Design review of the part built by this model. Coordinates are the model's own, in mm. Face numbers are marked on the shaded views. A direction names the side the tool comes from. Give positions to 0.01 mm unless a question says otherwise; leave off trailing zeros. Write each loop counter-clockwise with the first axis right and the second up, starting at its lowest first coordinate (ties: lowest second). Pieces come first, ordered by that corner, then holes. Notation, with made-up numbers: (55.25, -25.75) - (108.25, -25.75) arc R26 cw to (108.25, -5.75) - close; hole circle Ø11 at (16.5, -13.5). An arc over 180 degrees is marked (long way). Use a Markdown table: item, result. Add a question column.
```python
from build123d import *

# Parameters (mm, degrees)
F1_DEPTH = 101.6
F2_R     = 12.7
F3_DEPTH = 177.8
F4_R     = 7.9375
F4_R_2   = 6.35
F5_DEPTH = 177.8


with BuildPart() as f1:
    # F0 (on Front) → F1 (new body)
    with BuildSketch(Plane.XZ):
        with BuildLine():
            Line((-66.675, 136.525), (-66.675, 0))
            Line((-66.675, 0), (-60.325, 0))
            Line((-60.325, 0), (-60.325, 136.525))
            ThreePointArc((-60.325, 136.525), (-57.535192, 143.260192), (-50.8, 146.05))
            Line((-50.8, 146.05), (50.8, 146.05))
            ThreePointArc((50.8, 146.05), (57.535192, 143.260192), (60.325, 136.525))
            Line((60.325, 136.525), (60.325, 0))
            Line((60.325, 0), (66.675, 0))
            Line((66.675, 0), (66.675, 136.525))
            ThreePointArc((66.675, 136.525), (62.02532, 147.75032), (50.8, 152.4))
            Line((50.8, 152.4), (-50.8, 152.4))
            ThreePointArc((-50.8, 152.4), (-62.02532, 147.75032), (-66.675, 136.525))
        make_face()
    extrude(amount=F1_DEPTH)

    # F2 (on face) → F3 (join)
    with BuildSketch(Plane.XY.offset(152.4)):
        with Locations((0, -50.8)):
            Circle(F2_R)
    extrude(amount=F3_DEPTH)

    # F4 (on face) → F5 (cut)
    with BuildSketch(Plane.YZ.offset(66.675)):
        with BuildLine():
            Line((-101.6, 131.336227), (-101.6, 0))
            Line((-101.6, 0), (-25.4, 0))
            ThreePointArc((-25.4, 0), (-38.346191, 3.546942), (-47.676682, 13.197154))
            ThreePointArc((-47.676682, 13.197154), (-47.876619, 13.569464), (-48.070335, 13.945048))
            Line((-48.070335, 13.945048), (-94.291548, 101.759887))
            ThreePointArc((-94.291548, 101.759887), (-99.745816, 116.103258), (-101.6, 131.336227))
        make_face()
        with BuildLine():
            ThreePointArc((-48.070335, 13.945048), (-47.876619, 13.569464), (-47.676682, 13.197154))
            Line((-47.676682, 13.197154), (-48.070335, 13.945048))
        make_face()
        with Locations((-25.4, 25.4)):
            Circle(F4_R)
        with Locations((-50.8, 316.940695)):
            Circle(F4_R_2)
        with BuildLine():
            ThreePointArc((0, 25.4), (-7.439488, 7.439488), (-25.4, 0))
            Line((-25.4, 0), (0, 0))
            Line((0, 0), (0, 25.4))
        make_face()
    extrude(amount=-F5_DEPTH, mode=Mode.SUBTRACT)


solid = f1.part
```
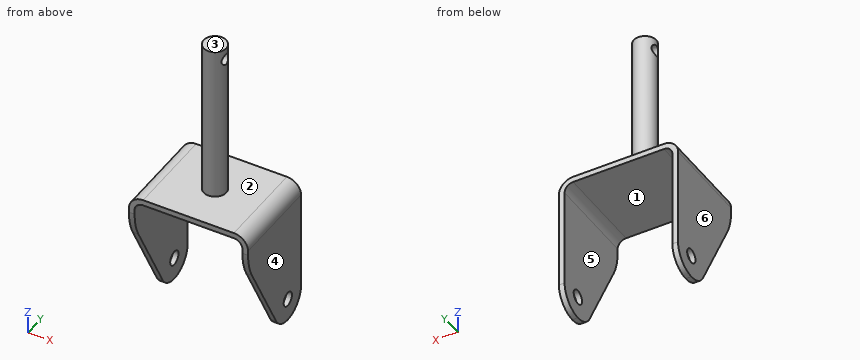
(1) Add section B-B (z = 67). State the section outline as (x, y) points (3 decimals), and give its area (3 significant figures).
(2) Mouldability with a two-part tool opening along X and no side actions: class the marked faces 4, 5 and 6 as +X half, -X half, draft (parallel to the pull), parting line (faces both ways), or undercut.
(3) Insertion check: pin 1 (14.5 mm diameter, centred on y = -50.8, z = 316.94, fed in from +X); pin 2 (4 mm diameter, centred on x = 6, y = -51, fed in from -Z); pin 3 (9.5 mm diameter, centred on y = -25.4, z = 25.4, fed in from +X); pin 4 (5 mm diameter, centred on y = -37.5, z = 171.5, fed in from +X). Each pin has a flat end and moves straight along its axis. Give the tip position at first contact, or say it passes through.
(4) Add section C-C (x = 46). State the section outline as (y, z) points.
(5) Tool access review of the marked faces 1, 2 and 3: name each direction out of +Z, -Z, +X, -X, +Y, -Y from which nothing blocks a thin tool from reaching the whole face with its end or side.
(6) Add section D-D (z = 278). State the section outline as (x, y) points, and give its area (3 significant figures).
(7) For line 1 along Z through (x, y) = (-5, -50.8); line 2 along X through (y, z) = (-15, 108) (3 decimals); line 3 along Z through (x, y) = (31.5, -91), list the stretches that pass through material, from the lowest coordinate up.
(8) Add section A-A (x = 2). State the section outline as (y, z) points, and give its area (3 significant figures).
Answers follow:
| question | item | result |
|---|---|---|
| 1 | outline | (-66.675, -75.996) - (-60.325, -75.996) - (-60.325, 0) - (-66.675, 0) - close; (60.325, -75.996) - (66.675, -75.996) - (66.675, 0) - (60.325, 0) - close |
| 1 | area | 965 mm^2 |
| 2 | face 4 | +X half |
| 2 | face 5 | undercut |
| 2 | face 6 | -X half |
| 3 | pin 1 | x = 12.7 |
| 3 | pin 2 | z = 146.05 |
| 3 | pin 3 | through |
| 3 | pin 4 | x = 6.68 |
| 4 | outline | (-101.6, 146.05) - (0, 146.05) - (0, 152.4) - (-101.6, 152.4) - close |
| 5 | face 1 | -Z, +Y, -Y |
| 5 | face 2 | +Z |
| 5 | face 3 | +Z, +X, -X, +Y, -Y |
| 6 | outline | circle Ø25.4 at (0, -50.8) |
| 6 | area | 507 mm^2 |
| 7 | line 1 | 146.05 to 310.59, 323.29 to 330.2 |
| 7 | line 2 | -66.675 to -60.325, 60.325 to 66.675 |
| 7 | line 3 | 146.05 to 152.4 |
| 8 | outline | (-101.6, 146.05) - (0, 146.05) - (0, 152.4) - (-38.26, 152.4) - (-38.26, 330.2) - (-63.34, 330.2) - (-63.34, 152.4) - (-101.6, 152.4) - close; hole circle Ø12.7 at (-50.8, 316.94) |
| 8 | area | 4,980 mm^2 |
